```python
from build123d import *

# Parameters (mm, degrees)
SKETCH1_W           = 80.264
SKETCH1_H           = 158.75
BOSS_EXTRUDE1_DEPTH = 3.048
SKETCH2_W           = 80.264
SKETCH2_H           = 158.75
BOSS_EXTRUDE2_DEPTH = 10.414
FILLET2_R           = 7.62
BOSS_EXTRUDE3_START = -1.27
BOSS_EXTRUDE3_DEPTH = 1.27
CUT_EXTRUDE1_DEPTH  = 179.39590141
CUT_EXTRUDE2_DEPTH  = 10.16
SKETCH6_W           = 19.304
SKETCH6_H           = 6.35
CUT_EXTRUDE4_DEPTH  = 3.81
SKETCH7_W           = 44.45
SKETCH7_H           = 6.35
CUT_EXTRUDE5_DEPTH  = 179.39590141


with BuildPart() as part:
    # Sketch1 → Boss-Extrude1 (new body)
    with BuildSketch(Plane(origin=(0, 0, 0), x_dir=(1, 0, 0), z_dir=(0, 1, 0))):
        with Locations((40.132, -79.375)):
            Rectangle(SKETCH1_W, SKETCH1_H)
    extrude(amount=BOSS_EXTRUDE1_DEPTH)

    # Sketch2 → Boss-Extrude2 (add)
    with BuildSketch(Plane(origin=(0, 3.048, 0), x_dir=(1, 0, 0), z_dir=(0, 1, 0))):
        with Locations((40.132, -79.375)):
            Rectangle(SKETCH2_W, SKETCH2_H)
        with BuildLine():
            Line((11.43, -3.81), (68.834, -3.81))
            ThreePointArc((68.834, -3.81), (74.222153673, -6.041846327), (76.454, -11.43))
            Line((76.454, -11.43), (76.454, -147.32))
            ThreePointArc((76.454, -147.32), (74.222153673, -152.708153673), (68.834, -154.94))
            Line((68.834, -154.94), (11.43, -154.94))
            ThreePointArc((11.43, -154.94), (6.041846327, -152.708153673), (3.81, -147.32))
            Line((3.81, -147.32), (3.81, -11.43))
            ThreePointArc((3.81, -11.43), (6.041846327, -6.041846327), (11.43, -3.81))
        make_face(mode=Mode.SUBTRACT)
    extrude(amount=BOSS_EXTRUDE2_DEPTH)

    # Fillet2
    fillet2_edges = [part.edges().sort_by_distance(p)[0] for p in [
        (0, 6.731, 0),
        (80.264, 6.731, 0),
        (80.264, 6.731, 158.75),
        (0, 6.731, 158.75),
    ]]
    fillet(fillet2_edges, radius=FILLET2_R)

    # Sketch3 → Boss-Extrude3 (add)
    with BuildSketch(Plane(origin=(0, 13.462, 0), x_dir=(1, 0, 0), z_dir=(0, 1, 0)).offset(BOSS_EXTRUDE3_START)):
        with BuildLine():
            Line((11.43, -3.81), (68.834, -3.81))
            ThreePointArc((68.834, -3.81), (74.222153673, -6.041846327), (76.454, -11.43))
            Line((76.454, -11.43), (76.454, -147.32))
            ThreePointArc((76.454, -147.32), (74.222153673, -152.708153673), (68.834, -154.94))
            Line((68.834, -154.94), (11.43, -154.94))
            ThreePointArc((11.43, -154.94), (6.041846327, -152.708153673), (3.81, -147.32))
            Line((3.81, -147.32), (3.81, -11.43))
            ThreePointArc((3.81, -11.43), (6.041846327, -6.041846327), (11.43, -3.81))
        make_face()
        with BuildLine():
            Line((13.661846327, -6.041846327), (66.602153673, -6.041846327))
            ThreePointArc((66.602153673, -6.041846327), (71.990307345, -8.273692655), (74.222153673, -13.661846327))
            Line((74.222153673, -13.661846327), (74.222153673, -145.088153673))
            ThreePointArc((74.222153673, -145.088153673), (71.990307345, -150.476307345), (66.602153673, -152.708153673))
            Line((66.602153673, -152.708153673), (13.661846327, -152.708153673))
            ThreePointArc((13.661846327, -152.708153673), (8.273692655, -150.476307345), (6.041846327, -145.088153673))
            Line((6.041846327, -145.088153673), (6.041846327, -13.661846327))
            ThreePointArc((6.041846327, -13.661846327), (8.273692655, -8.273692655), (13.661846327, -6.041846327))
        make_face(mode=Mode.SUBTRACT)
    extrude(amount=BOSS_EXTRUDE3_DEPTH)

    # Sketch4 → Cut-Extrude1 (cut, through all)
    with BuildSketch(Plane.XZ):
        with BuildLine():
            Line((12.7, 148.59), (40.64, 148.59))
            ThreePointArc((40.64, 148.59), (42.436051224, 147.846051224), (43.18, 146.05))
            Line((43.18, 146.05), (43.18, 118.11))
            ThreePointArc((43.18, 118.11), (42.436051224, 116.313948776), (40.64, 115.57))
            Line((40.64, 115.57), (12.7, 115.57))
            ThreePointArc((12.7, 115.57), (10.903948776, 116.313948776), (10.16, 118.11))
            Line((10.16, 118.11), (10.16, 146.05))
            ThreePointArc((10.16, 146.05), (10.903948776, 147.846051224), (12.7, 148.59))
        make_face()
    extrude(amount=-CUT_EXTRUDE1_DEPTH, mode=Mode.SUBTRACT)

    # Sketch5 → Cut-Extrude2 (cut)
    with BuildSketch(Plane(origin=(80.264, 0, 0), x_dir=(0, 0, -1), z_dir=(1, 0, 0))):
        Polygon((-98.298, 0), (-101.6, 3.302), (-90.932, 3.302), (-94.234, 0), align=None)
        Polygon((-60.452, 0), (-57.15, 3.302), (-67.818, 3.302), (-64.516, 0), align=None)
        Polygon((-39.243, 3.302), (-35.941, 0), (-31.877, 0), (-28.575, 3.302), align=None)
    cut_extrude2 = extrude(amount=-CUT_EXTRUDE2_DEPTH, mode=Mode.SUBTRACT)

    # Mirror1: Cut-Extrude2 across plane
    add(cut_extrude2.mirror(Plane(origin=(40.132, 0, 0), x_dir=(0, 0, 1), z_dir=(1, 0, 0))), mode=Mode.SUBTRACT)

    # Sketch6 → Cut-Extrude4 (cut)
    with BuildSketch(Plane(origin=(0, 0, 0), x_dir=(-1, 0, 0), z_dir=(0, 0, -1))):
        with Locations((-40.132, 6.731)):
            Rectangle(SKETCH6_W, SKETCH6_H)
    extrude(amount=-CUT_EXTRUDE4_DEPTH, mode=Mode.SUBTRACT)

    # Sketch7 → Cut-Extrude5 (cut, through all)
    with BuildSketch(Plane.ZY):
        with Locations((111.125, 7.62)):
            Rectangle(SKETCH7_W, SKETCH7_H)
    extrude(amount=-CUT_EXTRUDE5_DEPTH, mode=Mode.SUBTRACT)


solid = part.part
```
Build history of the part. All positions in model axes, mm. A direction names the side the tool comes from. Give positions to 0.01 mm unless a question says otherwise; leave off trailing zeros. Order: outer loops, then holes, each group sorted by start corner. A loop starts at its lowest first (then second) coordinate and runs counter-clockwise, first axis right, second up. Notation, with made-up numbers: M 38,62.5 L 55,62.5 A18 cw 55,94.5 Z; hole C 42.25,65 d8. An arc over 180 degrees is marked long. Write item = value, one per line. Start each with the question number.
(1) Two-plate mould, pull along Z, no slides. Class faces 1 (the flat face through (40, 7, 158.75)), 2 (the cylindrical face through (78.1, 6.6, 2.3)), 3 (the flat face through (76.454, 8, 63)), 4 (the flat face through (78, 4.445, 111)): released by +Z, released by -Z, zero draft, split by the parting line, or undercut.
(2) Probe L1, parallel to X at y = 3, z = 139.5; L2, parallel to Z at x = 18.5, y = 6; L3, parallel to Z at x = 31, y = 2.75. List the from-to ranges inside material, lowest first. Write a range as [from, to].
(3) Slice it at A-A on x = 32. Write the cut outline in (y, z), plus the area to 3 significant figures.
(4) Slice it at C-C on x = 17. Write the cut outline in (y, z).
(5) Slice it at D-D on z = 113. Write the cut outline in (x, y) (3 decimals).
(6) Pin check, flat tips, straight feed: pin 1 Ø3 at (x, y) = (77.5, 6.5) entering from +Z; pin 2 Ø22 at (x, z) = (32, 58.5) entering from +Y; pin 3 Ø1.5 at (y, z) = (2, 97.5) entering from -X. Stop position of each tip, or through.
(7) Slice it at B-B on z = 140. Write the cut outline in (x, y), plus the area to 3 significant figures.
(8) Which spindle directions (+Z, -Z, +X, -X, +Y, -Y) get a long thin tool onto all of the face, cutting with end or side? Do faces 5 (the flat face through (10.16, 2, 34)), 6 (the cylindrical face through (5.983, 7.556, 6.101)), 7 (the flat face through (78, 8, 133.35)), 8 (the flat face through (26, 2, 148.59)), 9 (the cylindrical face through (8.215, 12.818, 8.333)). Say none if no direction does.
Responses:
q1.face_1 = released by +Z
q1.face_2 = released by -Z
q1.face_3 = undercut
q1.face_4 = undercut
q2.L1 = [0, 10.16], [43.18, 80.26]
q2.L2 = [0, 3.81], [154.94, 158.75]
q2.L3 = [0, 115.57], [148.59, 158.75]
q3.outline = M 0,0 L 3.56,0 L 3.56,3.81 L 3.05,3.81 L 3.05,115.57 L 0,115.57 Z; M 0,148.59 L 3.05,148.59 L 3.05,154.94 L 12.19,154.94 L 12.19,152.71 L 13.46,152.71 L 13.46,158.75 L 0,158.75 Z; M 9.91,0 L 13.46,0 L 13.46,6.04 L 12.19,6.04 L 12.19,3.81 L 9.91,3.81 Z
q3.area = 444 mm2
q4.outline = M 0,0 L 13.46,0 L 13.46,6.04 L 12.19,6.04 L 12.19,3.81 L 3.05,3.81 L 3.05,115.57 L 0,115.57 Z; M 0,148.59 L 3.05,148.59 L 3.05,154.94 L 12.19,154.94 L 12.19,152.71 L 13.46,152.71 L 13.46,158.75 L 0,158.75 Z
q5.outline = M 0,0 L 80.264,0 L 80.264,4.445 L 76.454,4.445 L 76.454,3.048 L 3.81,3.048 L 3.81,4.445 L 0,4.445 Z; M 0,10.795 L 3.81,10.795 L 3.81,12.192 L 6.042,12.192 L 6.042,13.462 L 0,13.462 Z; M 74.222,12.192 L 76.454,12.192 L 76.454,10.795 L 80.264,10.795 L 80.264,13.462 L 74.222,13.462 Z
q6.pin_1 = 157.97
q6.pin_2 = 3.05
q6.pin_3 = 10.16
q7.outline = M 0,0 L 10.16,0 L 10.16,3.05 L 3.81,3.05 L 3.81,12.19 L 6.04,12.19 L 6.04,13.46 L 0,13.46 Z; M 43.18,0 L 80.26,0 L 80.26,13.46 L 74.22,13.46 L 74.22,12.19 L 76.45,12.19 L 76.45,3.05 L 43.18,3.05 Z
q7.area = 229 mm2
q8.face_5 = -X, +Y
q8.face_6 = none
q8.face_7 = +X, -X
q8.face_8 = +Y, -Y
q8.face_9 = +Y
